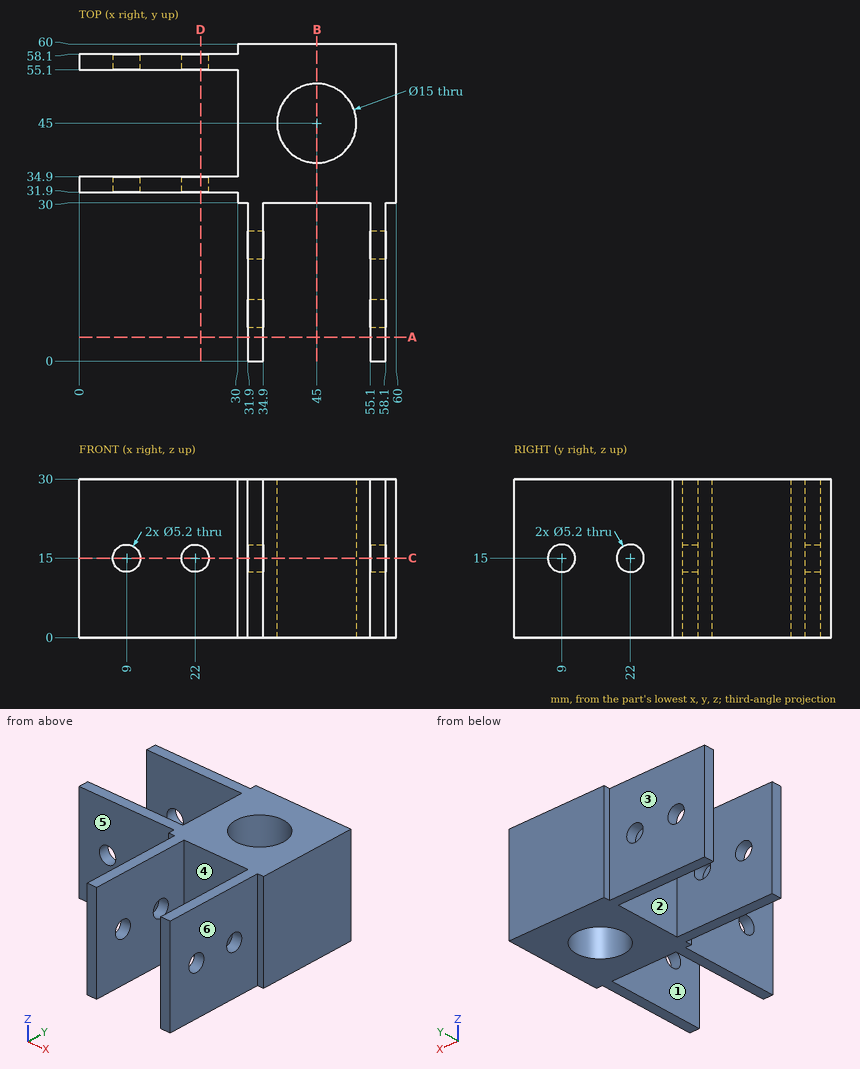
Design review of the part shown in the three views and the two pictorial views. Dimensions are in mm from the part's minimum x, y and z. A direction names the side the tool comes from. Round coordinates to 2 decimals unless told otherwise and drop trailing zeros. Order: outer loops, then holes, each group sorted by start corner. A loop starts at its lowest first (then second) coordinate and runs counter-clockwise, first axis right, second up.
(1) Take a section at C-C, the plane z = 15. Count the separate pieces of the cut face and the enclosed holes in it, plus the area to 3 significant figures.
Working result:
separate pieces: 9
enclosed holes: 1
area: 958 mm2
(2) Take a section at B-B, the plane x = 45. State the section outline as (y, z) points, plus the area to 3 significant figures.
Working result:
outline: (30, 0) - (37.5, 0) - (37.5, 30) - (30, 30) - close; (52.5, 0) - (60, 0) - (60, 30) - (52.5, 30) - close
area: 450 mm2
(3) For P1, Ø5, axis at x = 49, y = 38.5, coming from the -Z side; P2, Ø0.9, axis at y = 59, z = 20, coming from the -X side; P3, Ø9, axis at x = 11, z = 19, coming from the -Y side; P4, Ø1, axis at x = 54, z = 15, coming from the -Y side, all flat-tipped, find the tip position at first contact; note any pin that passes through.
Working result:
P1: stops at z = 0
P2: stops at x = 30
P3: stops at y = 31.9
P4: stops at y = 30
(4) Tool access review of the marked faces 1, 2 and 3: name each direction out of +Z, -Z, +X, -X, +Y, -Y from which nothing blocks a thin tool from reaching the whole face with its end or side.
Working result:
face 1: +Z, -Z, -Y
face 2: +Z, -Z, -X
face 3: +Z, -Z, -X, +Y
(5) Mouldability with a two-part tool opening along X and no side actions: class the marked faces 4, 5 and 6 as released by +X, released by -X, zero draft, split by the parting line, or undercut.
Working result:
face 4: undercut
face 5: zero draft
face 6: released by +X
(6) Wall thickness on L1, parallel to X at y = 56.5, z = 15.25; L2, parallel to Y at x = 6, z = 18.75: over which ranges is each line inside the solid? List them lowest first.
Working result:
L1: x = 0 to 6.41, 11.59 to 19.41, 24.59 to 60
L2: y = 31.9 to 34.9, 55.1 to 58.1
(7) Take a section at D-D, the plane x = 23. State the section outline as (y, z) points, plus the area to 3 significant figures.
Working result:
outline: (31.9, 0) - (34.9, 0) - (34.9, 12.6) - (31.9, 12.6) - close; (31.9, 17.4) - (34.9, 17.4) - (34.9, 30) - (31.9, 30) - close; (55.1, 0) - (58.1, 0) - (58.1, 12.6) - (55.1, 12.6) - close; (55.1, 17.4) - (58.1, 17.4) - (58.1, 30) - (55.1, 30) - close
area: 151 mm2
(8) Take a section at A-A, the plane y = 4.5. State the section outline as (x, z) points, plus the area to 3 significant figures.
Working result:
outline: (31.9, 0) - (34.9, 0) - (34.9, 30) - (31.9, 30) - close; (55.1, 0) - (58.1, 0) - (58.1, 30) - (55.1, 30) - close
area: 180 mm2
